Source: three-view drawing plus pictorial views. Frame: mm from the lowest corner of the part. Give positions to 0.01 mm unless a question says otherwise; leave off trailing zeros. Write each loop counter-clockwise with the first axis right and the second up, starting at its lowest first coordinate (ties: lowest second). Pieces come first, ordered by that corner, then holes.
Q1. Cut plane D-D on x = 10.5. Return the cut outline in (y, z).
Q2. Pin query (flat end, axial travel): pin 1 (5 mm diameter, centred on x = 42.5, y = 4, fed in from +Z) (1 decimal); pin 2 (1 mm diameter, centred on y = 8.5, z = 15, fed in from +X); pin 3 (6 mm diameter, centred on x = 13.5, y = 7.5, fed in from -Z); pin 4 (3 mm diameter, centred on x = 2.58, z = 25.57, fed in from -Y). Return the tip coordinate at first contact, or that it passes through.
Q3. Line query: L1, parallel to X at y = 5.5, z = 25 (1 decimal); L2, parallel to X at y = 0.5, z = 3 (1 decimal); L3, parallel to X at y = 4.5, z = 11 (1 decimal). Output: solid intervals per line, ascending.
Q4. Cut plane C-C on y = 7. Return the cut outline in (x, z) (1 decimal).
Q5. Cut plane B-B on x = 3. Return the cut outline in (y, z).
Q6. Draft query along X for the marked faces 1, 2 and 3. Return one class per face: pulls with the +X half, pulls with the -X half, needs draft (parallel to the pull), parting line crosses it, or undercut.
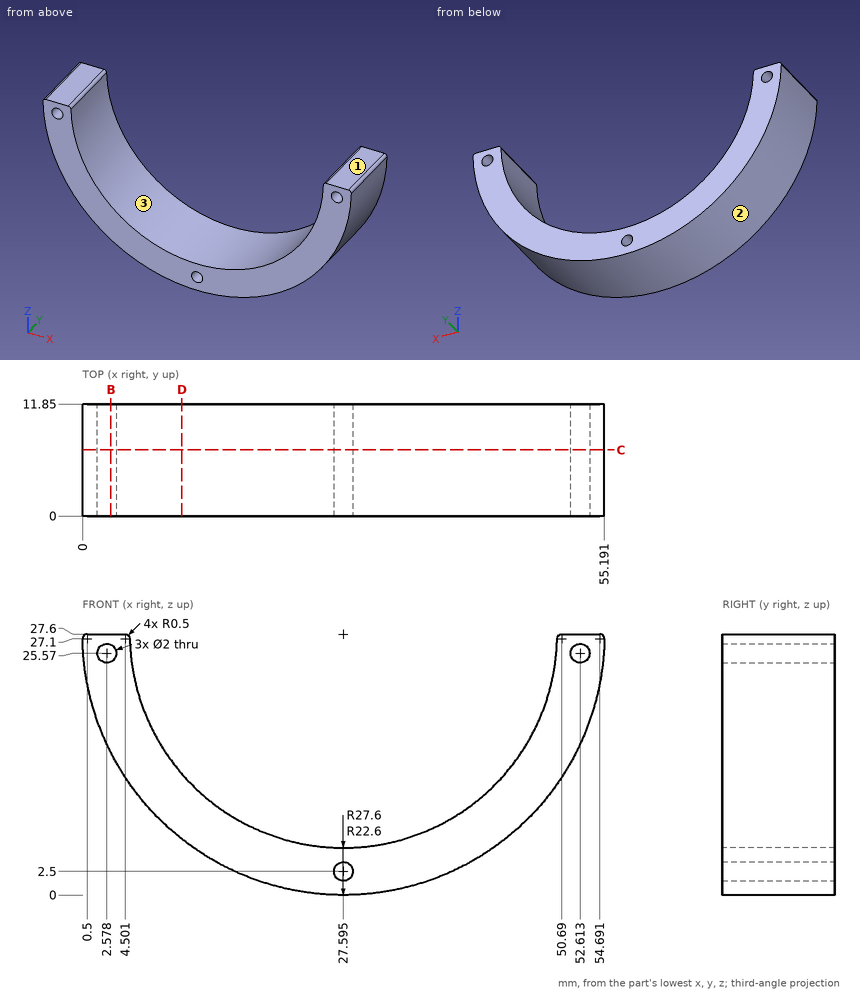
Data:
1. outline: (0, 5.93) - (11.85, 5.93) - (11.85, 12.82) - (0, 12.82) - close
2. pin 1: stops at z = 13.2
2. pin 2: stops at x = 52.4
2. pin 3: stops at z = 2.33
2. pin 4: stops at y = 0
3. L1: x = 0.1 to 1.8, 3.4 to 5.1, 50 to 51.8, 53.4 to 55.1
3. L2: x = 15.1 to 26.7, 28.5 to 40.1
3. L3: x = 5.5 to 12.3, 42.9 to 49.6
4. outline: (0, 27.1) arc R27.6 ccw to (55.2, 27.1) arc R0.5 ccw to (54.7, 27.6) - (50.7, 27.6) arc R0.5 ccw to (50.2, 27.1) arc R22.6 cw to (5, 27.1) arc R0.5 ccw to (4.5, 27.6) - (0.5, 27.6) arc R0.5 ccw to start; hole circle Ø2 at (2.6, 25.6); hole circle Ø2 at (27.6, 2.5); hole circle Ø2 at (52.6, 25.6)
5. outline: (0, 15.08) - (11.85, 15.08) - (11.85, 24.66) - (0, 24.66) - close; (0, 26.48) - (11.85, 26.48) - (11.85, 27.6) - (0, 27.6) - close
6. face 1: needs draft
6. face 2: parting line crosses it
6. face 3: undercut
